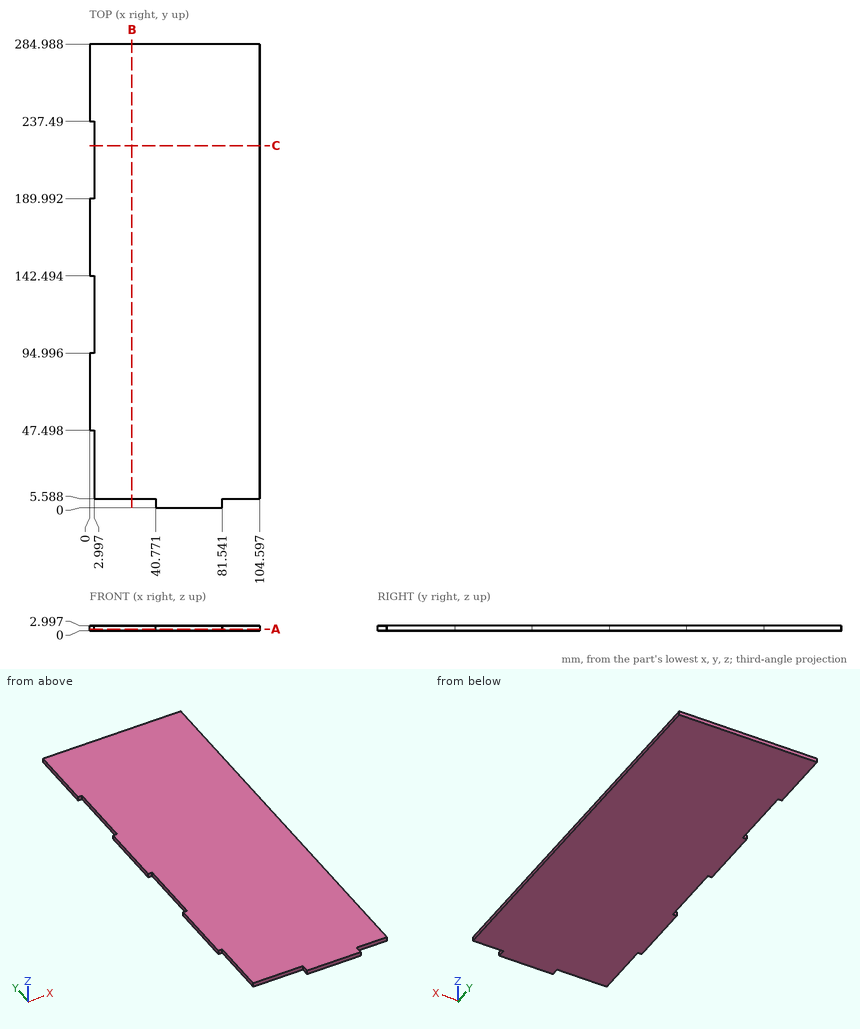
Geometry: see drawing. Coordinates: mm, zero at the bounding-box minimum. Round coordinates to 2 decimals unless told otherwise and drop trailing zeros. Loops run counter-clockwise (first coordinate to the right, second up) from the corner with the lowest first, then second, coordinate; pieces in that order, holes last. Notation, with made-up numbers: M 14.5,72.5 L 25.5,72.5 A19 cw 25.5,80.5 Z; hole C -10,26 d5. An arc over 180 degrees is marked long. Use a Markdown table: item, result. Add a question column.
1. Contact query for flat-ended pins moving along their axis: P1, Ø1, axis at x = 19, y = 81, coming from the -Z side; P2, Ø1, axis at y = 130, z = 2.5, coming from the -X side; P3, Ø1.5, axis at x = 1, z = 1.5, coming from the -Y side. Output: stop coordinate, or through.
2. Section query B-B on x = 26. Return the cut outline in (y, z).
3. Line query: line 1 (X direction, y = 230, z = 1.05); line 2 (Y direction, x = 95, z = 1.3). Output: solid intervals per line, ascending.
4. Section query A-A on z = 0.9. Return the cut outline in (x, y).
5. Section query C-C on y = 222.5. Return the cut outline in (x, z).
Reported:
| question | item | result |
|---|---|---|
| 1 | P1 | stops at z = 0 |
| 1 | P2 | stops at x = 3 |
| 1 | P3 | stops at y = 47.5 |
| 2 | outline | M 5.59,0 L 284.99,0 L 284.99,3 L 5.59,3 Z |
| 3 | line 1 | x = 3 to 104.6 |
| 3 | line 2 | y = 5.59 to 284.99 |
| 4 | outline | M 0,47.5 L 3,47.5 L 3,5.59 L 40.77,5.59 L 40.77,0 L 81.54,0 L 81.54,5.59 L 104.6,5.59 L 104.6,284.99 L 0,284.99 L 0,237.49 L 3,237.49 L 3,189.99 L 0,189.99 L 0,142.49 L 3,142.49 L 3,95 L 0,95 Z |
| 5 | outline | M 3,0 L 104.6,0 L 104.6,3 L 3,3 Z |
